Source: three-view drawing plus pictorial views. Frame: mm from the lowest corner of the part. Round coordinates to 2 decimals unless told otherwise and drop trailing zeros. Loops run counter-clockwise (first coordinate to the right, second up) from the corner with the lowest first, then second, coordinate; pieces in that order, holes last. Notation, with made-up numbers: (-15.75, 89.5) -> (33.25, 89.5) arc R25 cw to (33.25, 101.5) -> close; hole circle Ø10 at (60.25, -28). An arc over 180 degrees is marked (long way). Answer in a Markdown table with one row per item.
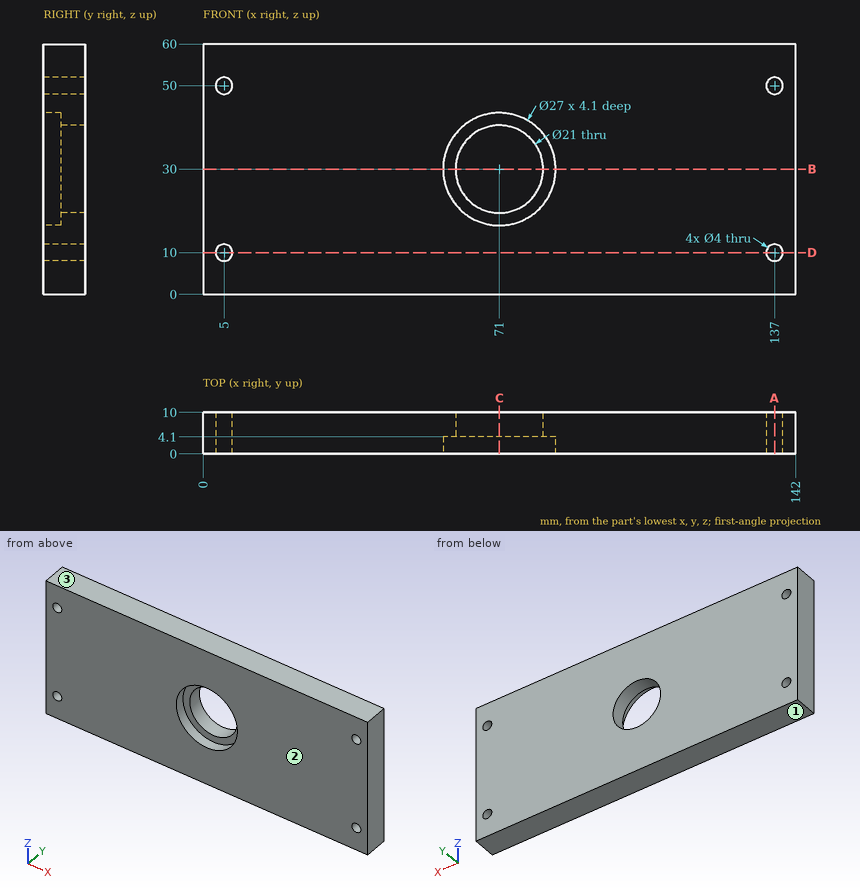
Item 1: Cut plane D-D (z = 10). Output: boundary loops of the cut face in (x, y), then the cut area to 3 significant figures.
Answer:
| item | result |
|---|---|
| outline | (0, 0) -> (3, 0) -> (3, 10) -> (0, 10) -> close; (7, 0) -> (135, 0) -> (135, 10) -> (7, 10) -> close; (139, 0) -> (142, 0) -> (142, 10) -> (139, 10) -> close |
| area | 1,340 mm² |
Item 2: Draft query along Z for the marked faces 1, 2 and 3. Return one class per face: pulls with the +Z half, pulls with the -Z half, needs draft (parallel to the pull), parting line crosses it, or undercut.
Answer:
| item | result |
|---|---|
| face 1 | pulls with the -Z half |
| face 2 | needs draft |
| face 3 | pulls with the +Z half |
Item 3: Cut plane A-A (x = 137). Output: boundary loops of the cut face in (y, z), then the cut area to 3 significant figures.
Answer:
| item | result |
|---|---|
| outline | (0, 0) -> (10, 0) -> (10, 8) -> (0, 8) -> close; (0, 12) -> (10, 12) -> (10, 48) -> (0, 48) -> close; (0, 52) -> (10, 52) -> (10, 60) -> (0, 60) -> close |
| area | 520 mm² |
Item 4: Line query: probe 1 along Z at (x, y) = (5, 4.25); probe 2 along Z at (x, y) = (71, 3.25); probe 3 along X at (y, z) = (0.5, 49.5). Output: solid intervals per line, ascending. Write a range as [from, to].
Answer:
| item | result |
|---|---|
| probe 1 | z = [0, 8], [12, 48], [52, 60] |
| probe 2 | z = [0, 16.5], [43.5, 60] |
| probe 3 | x = [0, 3.06], [6.94, 135.06], [138.94, 142] |
Item 5: Cut plane C-C (x = 71). Output: boundary loops of the cut face in (y, z), then the cut area to 3 significant figures.
Answer:
| item | result |
|---|---|
| outline | (0, 0) -> (10, 0) -> (10, 19.5) -> (4.1, 19.5) -> (4.1, 16.5) -> (0, 16.5) -> close; (0, 43.5) -> (4.1, 43.5) -> (4.1, 40.5) -> (10, 40.5) -> (10, 60) -> (0, 60) -> close |
| area | 365 mm² |
Item 6: Cut plane B-B (z = 30). Output: boundary loops of the cut face in (x, y), then the cut area to 3 significant figures.
Answer:
| item | result |
|---|---|
| outline | (0, 0) -> (57.5, 0) -> (57.5, 4.1) -> (60.5, 4.1) -> (60.5, 10) -> (0, 10) -> close; (81.5, 4.1) -> (84.5, 4.1) -> (84.5, 0) -> (142, 0) -> (142, 10) -> (81.5, 10) -> close |
| area | 1,190 mm² |
